Job drawing, mm, ordinate dimensions from the low corner. One solid piece. A direction names the side the tool comes from. Give positions to 0.01 mm unless a question says otherwise; leave off trailing zeros. Order: outer loops, then holes, each group sorted by start corner. A loop starts at its lowest first (then second) coordinate and runs counter-clockwise, first axis right, second up. Notation, with made-up numbers: (-19.75, 12) - (-2.75, 12) arc R21 cw to (-2.75, 29) - close; hole circle Ø7 at (-35.75, -17.75). An arc over 180 degrees is marked (long way). Use one line per item in the form item = value. Start each with the question number.
1. Tool access for the marked faces 1 and 2: list every direction of +Z, -Z, +X, -X, +Y, -Y with a clear straight run to the whole face (end or side of a thin tool).
2. Band-saw the part on D-D, the plane z = 10. List the corners of the cut face in (x, y), plus the area to 3 significant figures.
3. Pull direction Y, two halves, no side cores. Call the marked faces 3, 4 and 5: +Y half, -Y half, draft (parallel to the pull), parting line (faces both ways), or undercut.
4. Drill centre lines: line 1 (X direction, y = 2.6, z = 10); line 2 (Z direction, x = 12, y = 21); line 3 (Z direction, x = 13, y = 7). Where is each one in solid material? Low to high.
5. Band-saw the part on B-B, the plane x = 21. List the corners of the cut face in (y, z), plus the area to 3 significant figures.
6. Band-saw the part on A-A, the plane z = 37. List the corners of the cut face in (x, y).
7. Band-saw the part on C-C, the plane y = 2.5. List the corners of the cut face in (x, z).
8. Pin check, flat tips, straight feed: P1, Ø7, axis at x = 27, y = 17, coming from the -Z side; P2, Ø6, axis at x = 35, z = 10, coming from the +Y side; P3, Ø5.5, axis at y = 1.5, z = 9, coming from the -X side. Stop position of each tip, or through.
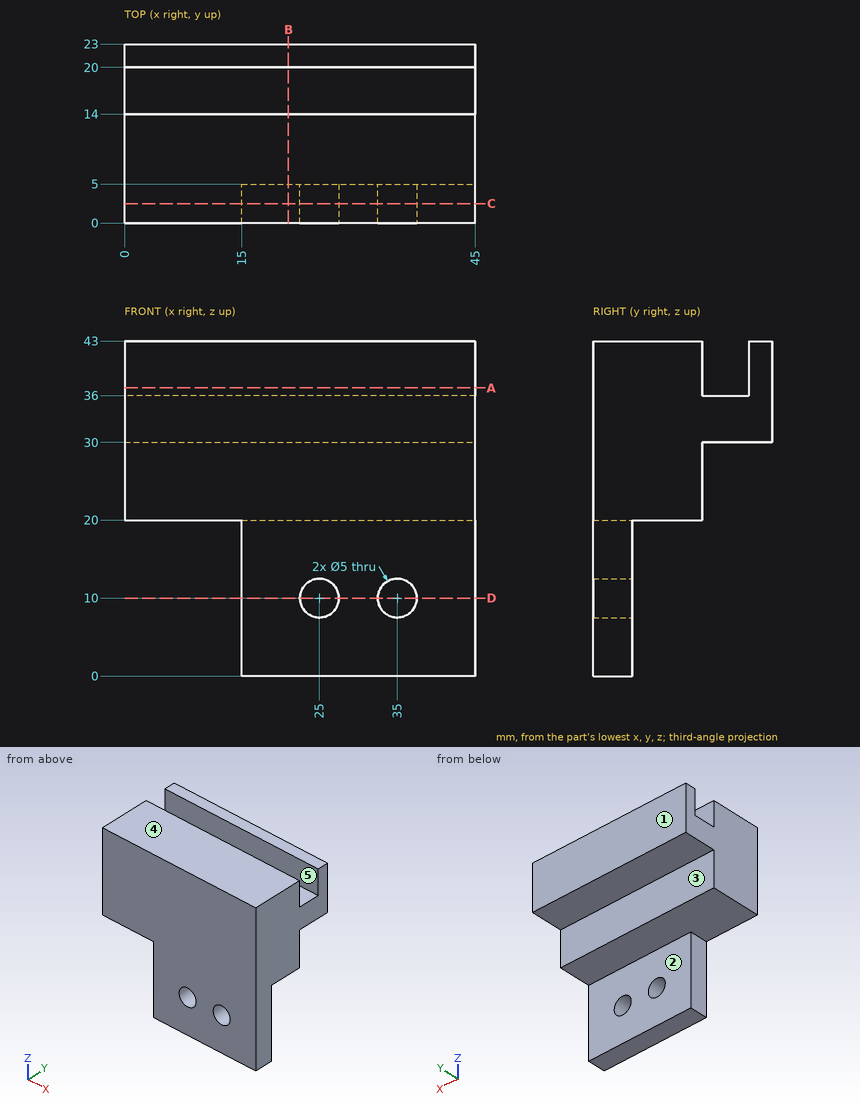
From the geometry:
q1.face_1 = +Z, -Z, +X, -X, +Y
q1.face_2 = -Z, +X, -X, +Y
q2.outline = (15, 0) - (22.5, 0) - (22.5, 5) - (15, 5) - close; (27.5, 0) - (32.5, 0) - (32.5, 5) - (27.5, 5) - close; (37.5, 0) - (45, 0) - (45, 5) - (37.5, 5) - close
q2.area = 100 mm²
q3.face_3 = +Y half
q3.face_4 = draft
q3.face_5 = undercut
q4.line_1 = 15 to 22.5, 27.5 to 32.5, 37.5 to 45
q4.line_2 = 30 to 43
q4.line_3 = 20 to 43
q5.outline = (0, 0) - (5, 0) - (5, 20) - (14, 20) - (14, 30) - (23, 30) - (23, 43) - (20, 43) - (20, 36) - (14, 36) - (14, 43) - (0, 43) - close
q5.area = 497 mm²
q6.outline = (0, 0) - (45, 0) - (45, 14) - (0, 14) - close; (0, 20) - (45, 20) - (45, 23) - (0, 23) - close
q7.outline = (0, 20) - (15, 20) - (15, 0) - (45, 0) - (45, 43) - (0, 43) - close; hole circle Ø5 at (25, 10); hole circle Ø5 at (35, 10)
q8.P1 = 20
q8.P2 = 5
q8.P3 = 15
